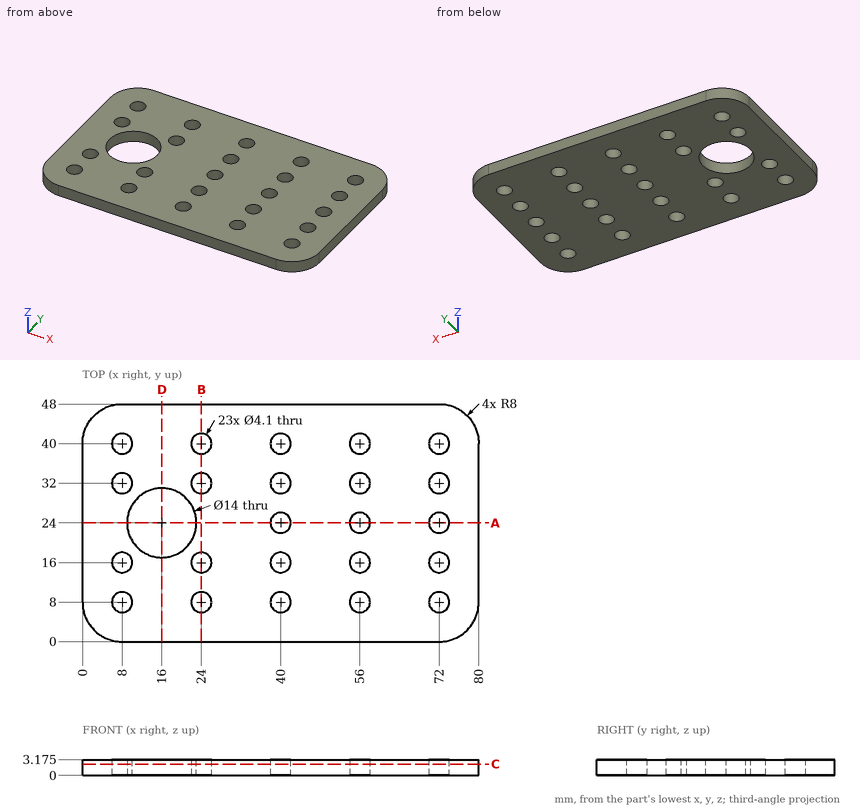
Study the drawing (mm; zero at the part's minimum x, y, z) and answer. Round coordinates to 2 decimals unless told otherwise and drop trailing zeros. Loops run counter-clockwise (first coordinate to the right, second up) from the corner with the lowest first, then second, coordinate; pieces in that order, holes last.
Q1. Section D-D, the plane x = 16 is taken. Determine the outline of the cut face in (y, z) (3 decimals), then the cut area to 3 significant figures.
Q2. Find the intervals of material crossed by line 1 (Y direction, x = 40, z = 1.5); line 2 (Y direction, x = 24, z = 1); line 3 (X direction, y = 32.5, z = 2.8), in increasing order.
Q3. Section A-A, the plane y = 24 is taken. Determine the outline of the cut face in (x, z) (3 decimals).
Q4. Given pin 1 Ø6.5 at (x, y) = (24, 40) entering from -Z; pin 2 Ø2.5 at (x, y) = (40, 40) entering from +Z, each flat-ended and moving along its own axis, determine where each tip first touches the part or whether it passes through.
Q5. Section B-B, the plane x = 24 is taken. Determine the outline of the cut face in (y, z) (3 decimals).
Q6. Section C-C, the plane z = 2.3 is taken. Count the separate pieces of the cut face and the enclosed holes in it, then the cut area to 3 significant figures.
Completed:
1. outline: (0, 0) - (17, 0) - (17, 3.175) - (0, 3.175) - close; (31, 0) - (48, 0) - (48, 3.175) - (31, 3.175) - close
1. area: 108 mm2
2. line 1: y = 0 to 5.95, 10.05 to 13.95, 18.05 to 21.95, 26.05 to 29.95, 34.05 to 37.95, 42.05 to 48
2. line 2: y = 0 to 5.95, 10.05 to 13.95, 18.05 to 29.95, 34.05 to 37.95, 42.05 to 48
2. line 3: x = 0 to 6.01, 9.99 to 22.01, 25.99 to 38.01, 41.99 to 54.01, 57.99 to 70.01, 73.99 to 80
3. outline: (0, 0) - (9, 0) - (9, 3.175) - (0, 3.175) - close; (23, 0) - (37.95, 0) - (37.95, 3.175) - (23, 3.175) - close; (42.05, 0) - (53.95, 0) - (53.95, 3.175) - (42.05, 3.175) - close; (58.05, 0) - (69.95, 0) - (69.95, 3.175) - (58.05, 3.175) - close; (74.05, 0) - (80, 0) - (80, 3.175) - (74.05, 3.175) - close
4. pin 1: stops at z = 0
4. pin 2: passes through
5. outline: (0, 0) - (5.95, 0) - (5.95, 3.175) - (0, 3.175) - close; (10.05, 0) - (13.95, 0) - (13.95, 3.175) - (10.05, 3.175) - close; (18.05, 0) - (29.95, 0) - (29.95, 3.175) - (18.05, 3.175) - close; (34.05, 0) - (37.95, 0) - (37.95, 3.175) - (34.05, 3.175) - close; (42.05, 0) - (48, 0) - (48, 3.175) - (42.05, 3.175) - close
6. separate pieces: 1
6. enclosed holes: 24
6. area: 3,330 mm2
